from build123d import *

# Parameters (mm, degrees)
SKETCH1_R            = 1.5
BOSS_EXTRUDE1_DEPTH  = 5
FILLET1_R            = 2
FILLET1_OF_MIRROR1_R = 2
SKETCH2_W            = 70
SKETCH2_H            = 97
CUT_EXTRUDE1_DEPTH   = 3
FILLET2_R            = 5


with BuildPart() as part:
    # Sketch1 → Boss-Extrude1 (new body)
    with BuildSketch(Plane(origin=(0, 0, 0), x_dir=(1, 0, 0), z_dir=(0, 1, 0))):
        Polygon((-52.164149312, -38.645247828), (-70, -25.247940817), (-70, 24.752308679), (-24.752308679, 70), (0, 70), (0, -30), (-38.851635079, -30), align=None)
        with Locations((-43.840620434, 43.840620434)):
            Circle(SKETCH1_R, mode=Mode.SUBTRACT)
        with Locations((-51.997575213, -33.767620171)):
            Circle(SKETCH1_R, mode=Mode.SUBTRACT)
        with Locations((-59.39696962, 28.284271247)):
            Circle(SKETCH1_R, mode=Mode.SUBTRACT)
        with Locations((-56.997575213, 33.73741674)):
            Circle(SKETCH1_R, mode=Mode.SUBTRACT)
        with Locations((-56.997575213, -31.26258326)):
            Circle(SKETCH1_R, mode=Mode.SUBTRACT)
        with Locations((-48.5, 40)):
            Circle(SKETCH1_R, mode=Mode.SUBTRACT)
        Polygon((-59.095959493, 22.1), (-57.095959493, 22.1), (-44.547727215, 34.648232278), (-40.5, 30.600505063), (-40.5, -23), (-48.796166422, -28.387593469), (-51, -23), (-55, -23), (-56.33662338, -29.883022962), (-65.5, -23), (-65.5, 22.181240867), (-62.33860018, 25.342640687), align=None, mode=Mode.SUBTRACT)
    boss_extrude1 = extrude(amount=BOSS_EXTRUDE1_DEPTH)

    # Fillet1
    fillet1_edges = [part.edges().sort_by_distance(p)[0] for p in [
        (-44.547727215, 2.5, -34.648232278),
        (-62.33860018, 2.5, -25.342640687),
        (-65.5, 2.5, -22.181240867),
        (-65.5, 2.5, 23),
        (-56.33662338, 2.5, 29.883022962),
        (-48.796166422, 2.5, 28.387593469),
        (-40.5, 2.5, 23),
        (-40.5, 2.5, -30.600505063),
    ]]
    fillet(fillet1_edges, radius=FILLET1_R)

    # Mirror1: Boss-Extrude1 across plane
    add(boss_extrude1.mirror(Plane(origin=(0, 5, 30), x_dir=(0, 0, 1), z_dir=(-1, 0, 0))))

    # Fillet1 of Mirror1
    fillet1_of_mirror1_edges = [part.edges().sort_by_distance(p)[0] for p in [
        (44.547727215, 2.5, -34.648232278),
        (62.33860018, 2.5, -25.342640687),
        (65.5, 2.5, -22.181240867),
        (65.5, 2.5, 23),
        (56.33662338, 2.5, 29.883022962),
        (48.796166422, 2.5, 28.387593469),
        (40.5, 2.5, 23),
        (40.5, 2.5, -30.600505063),
    ]]
    fillet(fillet1_of_mirror1_edges, radius=FILLET1_OF_MIRROR1_R)

    # Sketch2 → Cut-Extrude1 (cut)
    with BuildSketch(Plane(origin=(0, 0, 0), x_dir=(1, 0, 0), z_dir=(0, 1, 0))):
        with Locations((0, 21.5)):
            Rectangle(SKETCH2_W, SKETCH2_H)
    extrude(amount=CUT_EXTRUDE1_DEPTH, mode=Mode.SUBTRACT)

    # Fillet2
    fillet2_edges = [part.edges().sort_by_distance(p)[0] for p in [
        (-70, 2.5, -24.752308679),
        (-24.752308679, 4, -70),
        (-38.851635079, 2.5, 30),
        (-52.164149312, 2.5, 38.645247828),
        (-70, 2.5, 25.247940817),
        (70, 2.5, 25.247940817),
        (70, 2.5, -24.752308679),
        (24.752308679, 4, -70),
        (38.851635079, 2.5, 30),
        (52.164149312, 2.5, 38.645247828),
    ]]
    fillet(fillet2_edges, radius=FILLET2_R)


solid = part.part
Part model, mm, in its own coordinate system. A direction names the side the tool comes from. Coordinates: 2 decimals unless noted, no trailing zeros. Loops run counter-clockwise (first coordinate to the right, second up) from the corner with the lowest first, then second, coordinate; pieces in that order, holes last. Notation, with made-up numbers: (-37, 76.25) - (11, 76.25) arc R21 cw to (11, 87.25) - close; hole circle Ø4 at (-33.5, 75.5). An arc over 180 degrees is marked (long way). Write each question's results on one line, items separated by ' | '. Start each with the question number.
Q1. Probe line 1 along X through (y, z) = (2.25, -10); line 2 along X through (y, z) = (3.1, 3); line 3 along Z through (x, y) = (45, 1.5). List the from-to ranges inside material, lowest first.
Q2. Slice it at C-C on z = -40. Give the cut face in (x, y).
Q3. Slice it at B-B on x = 3. Give the cut face in (y, z).
Q4. Which spindle directions (+Z, -Z, +X, -X, +Y, -Y) get a long thin tool onto all of the face, cutting with end or side? Do faces 1 (the flat face through (-44.053, 2.465, 25.307)), 2 (the cylindrical face through (38.77, 2.54, 30.2)), 3 (the cylindrical face through (69.63, 2.54, -24.57)). Say none if no direction does.
Q5. Drop flat-ended pins along their axis: pin 1 Ø1.5 at (y, z) = (2, -24.5) entering from -X; pin 2 Ø1 at (x, z) = (-19, -13.5) entering from -Y; pin 3 Ø1 at (x, y) = (-58.5, 2) entering from +Z. Give the stop position or say it passes through.
Q6. Slice it at D-D on y = 1.95. Give the number of separate pieces and of enclosed holes in the cut face, and give its area (3 significant figures).
Q7. Slice it at A-A on z = 0. Give the cut face in (x, y).
Q8. Two-plate mould, pull along Z, no slides. Class faces 4 (the flat face through (0, 3, -22)), 5 (the cylindrical face through (58.188, 2.465, -32.825)), 6 (the cylindrical face through (-38.81, 2.54, 30.21)): +Z half, -Z half, draft (parallel to the pull), parting line (faces both ways), or undercut.
Answer:
1) line 1: x = -70 to -65.5, -40.5 to -35, 35 to 40.5, 65.5 to 70 | line 2: x = -70 to -65.5, -40.5 to 40.5, 65.5 to 70 | line 3: z = -49.75 to -44.79, -42.89 to -33.77, 25.92 to 33.99
2) outline: (-54.75, 0) - (-50, 0) - (-50, 5) - (-54.75, 5) - close; (-47, 0) - (-35, 0) - (-35, 3) - (35, 3) - (35, 0) - (47, 0) - (47, 5) - (-47, 5) - close; (50, 0) - (54.75, 0) - (54.75, 5) - (50, 5) - close
3) outline: (0, 27) - (3, 27) - (3, -70) - (5, -70) - (5, 30) - (0, 30) - close
4) face 1: +Y, -Y | face 2: +Z, +Y, -Y | face 3: -Z, +X, +Y, -Y
5) pin 1: stops at x = -69.88 | pin 2: stops at y = 3 | pin 3: stops at z = 34.26
6) separate pieces: 1 | enclosed holes: 14 | area: 2,720 mm2
7) outline: (-70, 0) - (-65.5, 0) - (-65.5, 5) - (-70, 5) - close; (-40.5, 0) - (-35, 0) - (-35, 3) - (35, 3) - (35, 0) - (40.5, 0) - (40.5, 5) - (-40.5, 5) - close; (65.5, 0) - (70, 0) - (70, 5) - (65.5, 5) - close
8) face 4: draft | face 5: undercut | face 6: +Z half
